from build123d import *

# Parameters (mm, degrees)
F1_DEPTH = 9


with BuildPart() as f1:
    # F0 (on Front) → F1 (new body)
    with BuildSketch(Plane.XZ):
        with BuildLine():
            Line((13, 0), (11, 0))
            ThreePointArc((11, 0), (10.695268783, -2.5712303784), (9.7979589711, -5))
            Line((9.7979589711, -5), (12, -5))
            ThreePointArc((12, -5), (12.747548784, -2.5495097568), (13, 0))
        make_face()
        with BuildLine():
            ThreePointArc((9.7979589711, 5), (10.695268783, 2.5712303784), (11, 0))
            Line((11, 0), (13, 0))
            ThreePointArc((13, 0), (12.747548784, 2.5495097568), (12, 5))
            Line((12, 5), (9.7979589711, 5))
        make_face()
        with BuildLine():
            ThreePointArc((5, 9.7979589711), (7.7781745931, 7.7781745931), (9.7979589711, 5))
            Line((9.7979589711, 5), (12, 5))
            ThreePointArc((12, 5), (9.1923881554, 9.1923881554), (5, 12))
            Line((5, 12), (5, 9.7979589711))
        make_face()
        with BuildLine():
            Line((12, -5), (9.7979589711, -5))
            ThreePointArc((9.7979589711, -5), (7.7781745931, -7.7781745931), (5, -9.7979589711))
            Line((5, -9.7979589711), (5, -12))
            ThreePointArc((5, -12), (9.1923881554, -9.1923881554), (12, -5))
        make_face()
        with BuildLine():
            Line((24.7979589711, 0), (13, 0))
            ThreePointArc((13, 0), (12.747548784, -2.5495097568), (12, -5))
            Line((12, -5), (24.7979589711, -5))
            Line((24.7979589711, -5), (24.7979589711, 0))
        make_face()
        with BuildLine():
            ThreePointArc((12, 5), (12.747548784, 2.5495097568), (13, 0))
            Line((13, 0), (24.7979589711, 0))
            Line((24.7979589711, 0), (24.7979589711, 5))
            Line((24.7979589711, 5), (12, 5))
        make_face()
        with BuildLine():
            ThreePointArc((0, 11), (2.5712303784, 10.695268783), (5, 9.7979589711))
            Line((5, 9.7979589711), (5, 12))
            ThreePointArc((5, 12), (2.5495097568, 12.747548784), (0, 13))
            Line((0, 13), (0, 11))
        make_face()
        with BuildLine():
            Line((5, -12), (5, -9.7979589711))
            ThreePointArc((5, -9.7979589711), (2.5712303784, -10.695268783), (0, -11))
            Line((0, -11), (0, -13))
            ThreePointArc((0, -13), (2.5495097568, -12.747548784), (5, -12))
        make_face()
        with BuildLine():
            Line((0, -13), (0, -11))
            ThreePointArc((0, -11), (-2.5712303784, -10.695268783), (-5, -9.7979589711))
            Line((-5, -9.7979589711), (-5, -12))
            ThreePointArc((-5, -12), (-2.5495097568, -12.747548784), (0, -13))
        make_face()
        with BuildLine():
            Line((-13, 0), (-11, 0))
            ThreePointArc((-11, 0), (-10.807426658, 2.0492752456), (-10.2364492669, 4.0267985307))
            Line((-10.2364492669, 4.0267985307), (-12.3606186574, 4.0267985307))
            ThreePointArc((-12.3606186574, 4.0267985307), (-12.8391596794, 2.0386217715), (-13, 0))
        make_face()
        with BuildLine():
            ThreePointArc((-9.2369293711, -5.9732014693), (-10.550028983, -3.1139827326), (-11, 0))
            Line((-11, 0), (-13, 0))
            ThreePointArc((-13, 0), (-12.6313904767, -3.073755785), (-11.5464654422, -5.9732014693))
            Line((-11.5464654422, -5.9732014693), (-9.2369293711, -5.9732014693))
        make_face()
        with BuildLine():
            ThreePointArc((-5, 9.7979589711), (-2.5712303784, 10.695268783), (0, 11))
            Line((0, 11), (0, 13))
            ThreePointArc((0, 13), (-2.5495097568, 12.747548784), (-5, 12))
            Line((-5, 12), (-5, 9.7979589711))
        make_face()
        Polygon((45.145274992, 0), (24.7979589711, 0), (24.7979589711, -5), (45.145274992, -13.2566292219), align=None)
        Polygon((24.7979589711, 5), (24.7979589711, 0), (45.145274992, 0), (45.145274992, 13.2566292219), align=None)
        with BuildLine():
            ThreePointArc((0, 13), (2.5495097568, 12.747548784), (5, 12))
            Line((5, 12), (5, 24.7979589711))
            Line((5, 24.7979589711), (0, 24.7979589711))
            Line((0, 24.7979589711), (0, 13))
        make_face()
        with BuildLine():
            Line((5, -24.7979589711), (5, -12))
            ThreePointArc((5, -12), (2.5495097568, -12.747548784), (0, -13))
            Line((0, -13), (0, -24.7979589711))
            Line((0, -24.7979589711), (5, -24.7979589711))
        make_face()
        with BuildLine():
            Line((-5, -12), (-5, -9.7979589711))
            ThreePointArc((-5, -9.7979589711), (-7.3708705026, -8.1651863441), (-9.2369293711, -5.9732014693))
            Line((-9.2369293711, -5.9732014693), (-11.5464654422, -5.9732014693))
            ThreePointArc((-11.5464654422, -5.9732014693), (-8.8049392269, -9.5641541816), (-5, -12))
        make_face()
        with BuildLine():
            Line((0, -24.7979589711), (0, -13))
            ThreePointArc((0, -13), (-2.5495097568, -12.747548784), (-5, -12))
            Line((-5, -12), (-5, -24.7979589711))
            Line((-5, -24.7979589711), (0, -24.7979589711))
        make_face()
        with BuildLine():
            Line((-12.3606186574, 4.0267985307), (-10.2364492669, 4.0267985307))
            ThreePointArc((-10.2364492669, 4.0267985307), (-8.1464053283, 7.3916223001), (-5, 9.7979589711))
            Line((-5, 9.7979589711), (-5, 12))
            ThreePointArc((-5, 12), (-9.5520026936, 8.8181202385), (-12.3606186574, 4.0267985307))
        make_face()
        with BuildLine():
            Line((-25.2364492669, 0), (-13, 0))
            ThreePointArc((-13, 0), (-12.8391596794, 2.0386217715), (-12.3606186574, 4.0267985307))
            Line((-12.3606186574, 4.0267985307), (-25.2364492669, 4.0267985307))
            Line((-25.2364492669, 4.0267985307), (-25.2364492669, 0))
        make_face()
        with BuildLine():
            ThreePointArc((-11.5464654422, -5.9732014693), (-12.6313904767, -3.073755785), (-13, 0))
            Line((-13, 0), (-25.2364492669, 0))
            Line((-25.2364492669, 0), (-25.2364492669, -0.9732014693))
            Line((-25.2364492669, -0.9732014693), (-25.2364492669, -5.9732014693))
            Line((-25.2364492669, -5.9732014693), (-11.5464654422, -5.9732014693))
        make_face()
        with BuildLine():
            ThreePointArc((-5, 12), (-2.5495097568, 12.747548784), (0, 13))
            Line((0, 13), (0, 24.7979589711))
            Line((0, 24.7979589711), (-5, 24.7979589711))
            Line((-5, 24.7979589711), (-5, 12))
        make_face()
        Polygon((45.145274992, 13.2566292219), (45.145274992, 0), (65.492591013, 0), (49.8166139769, 15.1521870403), align=None)
        Polygon((65.492591013, 0), (45.145274992, 0), (45.145274992, -13.2566292219), (49.8166139769, -15.1521870403), align=None)
        Polygon((0, 24.7979589711), (5, 24.7979589711), (13.9004829156, 46.4947918511), (0, 46.4947918511), align=None)
        Polygon((13.0237015361, -46.4836081518), (5, -24.7979589711), (0, -24.7979589711), (0, -46.4836081518), align=None)
        Polygon((0, -46.4836081518), (0, -24.7979589711), (-5, -24.7979589711), (-13.0237015361, -46.4836081518), (-1.1742307931, -46.4836081518), align=None)
        Polygon((-39.6632513358, 0), (-25.2364492669, 0), (-25.2364492669, 4.0267985307), (-47.5232979005, 12.7201679595), (-47.5232979005, 6.807), (-43.5932746181, 6.807), align=None)
        Polygon((-25.2364492669, -0.9732014693), (-25.2364492669, 0), (-39.6632513358, 0), (-43.5932746181, -6.807), (-47.5232979005, -6.807), (-47.5232979005, -12.7201679595), (-25.2364492669, -5.9732014693), align=None)
        Polygon((-5, 24.7979589711), (0, 24.7979589711), (0, 46.4947918511), (-13.9004829156, 46.4947918511), align=None)
        Polygon((0, 46.4947918511), (13.9004829156, 46.4947918511), (15.2472511326, 49.7778277503), (0, 66.8410263726), align=None)
        Polygon((14.3692514548, -50.1202244144), (13.0237015361, -46.4836081518), (0, -46.4836081518), (0, -65.8470422888), align=None)
        Polygon((0, -65.8470422888), (0, -46.4836081518), (-1.1742307931, -46.4836081518), (-13.0237015361, -46.4836081518), (-14.3692514548, -50.1202244144), align=None)
        Polygon((-13.9004829156, 46.4947918511), (0, 46.4947918511), (0, 66.8410263726), (-15.2472511326, 49.7778277503), align=None)
        Polygon((-47.5232979005, 6.807), (-47.5232979005, 12.7201679595), (-50.3905497057, 13.8385889439), (-69.8101465342, 0), (-55.3833444653, 0), (-51.4533211829, 6.807), align=None)
        Polygon((-51.0782389318, -13.7963662326), (-47.5232979005, -12.7201679595), (-47.5232979005, -6.807), (-51.4533211829, -6.807), (-55.3833444653, 0), (-69.8101465342, 0), align=None)
    extrude(amount=F1_DEPTH)


solid = f1.part
Here's how the part is built. I have some questions about the finished solid (model axes, mm). A direction names the side the tool comes from. Give positions to 0.01 mm unless a question says otherwise; leave off trailing zeros. Loops run counter-clockwise (first coordinate to the right, second up) from the corner with the lowest first, then second, coordinate; pieces in that order, holes last. Notation, with made-up numbers: (78.25, 7) -> (111.25, 7) arc R17 cw to (111.25, 15) -> close; hole circle Ø3 at (34.25, -28). An arc over 180 degrees is marked (long way). Answer as a JSON object with one key per item and string values. Group by question number.
Item 1: Imagine slicing it at A-A on y = -2. Give the number of separate pieces and of enclosed holes in the cut face, then the cut area to 3 significant figures.
Item 2: Thinking about a two-plate mould opening in Z: for faces 1 (the flat face through (-5, -4, 18)), 2 (the flat face through (-59.96, -4.44, 7.02)), 3 (the flat face through (57.545, -4.437, -7.682)), which applies, pulls with the +Z half, pulls with the -Z half, needs draft (parallel to the pull), parting line crosses it, or undercut?
Item 3: On a 3-axis mill with a long thin cutter (end or side, diameter ignored), from which of +Z, -Z, +X, -X, +Y, -Y can I reach the whole of each face in a straight line? I mean faces 4 (the flat face through (57.764, -4.437, 7.47)), 5 (the flat face through (-18, -4, -5.973)). Say none if no direction works.
Item 4: I need wall thicknesses on L1, parallel to X at y = -6, z = -2.5; L2, parallel to X at y = -0.5, z = -17; L3, parallel to X at y = -7, z = -2. Which ranges of each line are inside material? Lowest first, please.
Item 5: Will these pins go through, and if not, where does the flat tip stop? pin 1 (4.5 mm diameter, centred on y = -3.5, z = -17.5, fed in from -X); pin 2 (1 mm diameter, centred on y = -5, z = 32.5, fed in from -X); pin 3 (2.5 mm diameter, centred on x = -17.5, y = -5, fed in from -Z).
Item 6: Imagine slicing it at C-C on x = -21. Write out the boundary of the cut face in (y, z), then the cut area to 3 significant figures.
Item 7: Imagine slicing it at B-B on z = 20. Write out the boundary of the cut face in (x, y), then the cut area to 3 significant figures.
Answer list:
{
 "1": {"separate pieces": "1", "enclosed holes": "2", "area": "3,450 mm2"},
 "2": {"face 1": "undercut", "face 2": "pulls with the +Z half", "face 3": "pulls with the -Z half"},
 "3": {"face 4": "+Z, +X, +Y, -Y", "face 5": "+Y, -Y"},
 "4": {"L1": "x = -66.42 to -53.94, -41.11 to -10.71, 10.71 to 62.91", "L2": "x = -5 to 5", "L3": "x = -67.09 to -54.23, -40.82 to -10.82, 10.82 to 63.42"},
 "5": {"pin 1": "stops at x = -5", "pin 2": "stops at x = -8.36", "pin 3": "stops at z = -5.97"},
 "6": {"outline": "(-9, -5.97) -> (0, -5.97) -> (0, 4.03) -> (-9, 4.03) -> close", "area": "90.0 mm2"},
 "7": {"outline": "(-5, -9) -> (5, -9) -> (5, 0) -> (-5, 0) -> close", "area": "90.0 mm2"}
}
